Part print with two shaded views. Sizes in mm from the minimum x, y, z corner. Coordinates: 2 decimals unless noted, no trailing zeros. Loops run counter-clockwise (first coordinate to the right, second up) from the corner with the lowest first, then second, coordinate; pieces in that order, holes last. Notation, with made-up numbers: (-11.5, 9) - (27.5, 9) arc R15 ccw to (27.5, 29) - close; hole circle Ø2 at (72, 86). An arc over 180 degrees is marked (long way). Answer as CSV lines item,"result".
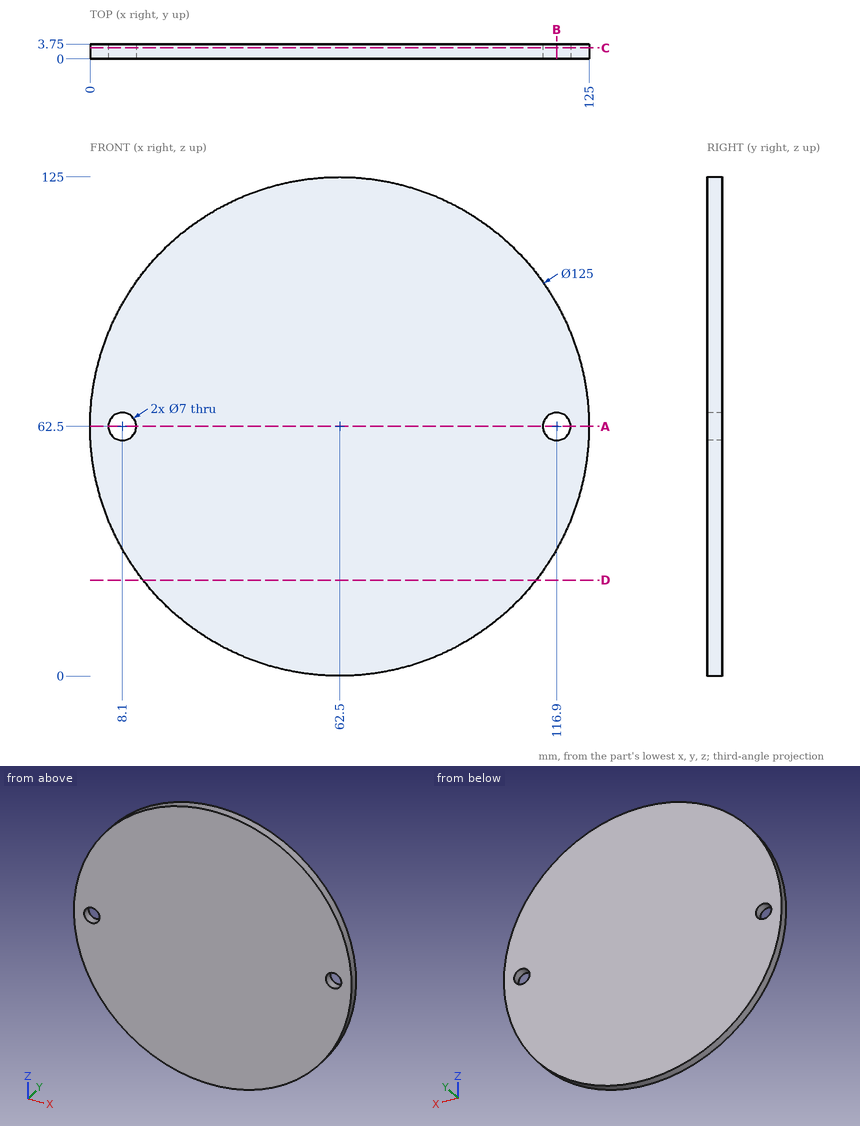
Q1. Saw through at C-C (y = 2.75). Give the cut face in (x, z).
Results:
outline,"circle Ø125 at (62.5, 62.5); hole circle Ø7 at (8.1, 62.5); hole circle Ø7 at (116.9, 62.5)"
Q2. Flat gauge pins, fed straight in: pin 1 (2 mm diameter, centred on y = 3, z = 29.5, fed in from +X); pin 2 (5.5 mm diameter, centred on x = 116.9, z = 62.5, fed in from -Y). Where does each tip first touch, or does it go through?
Results:
pin 1,"stops at x = 116.19"
pin 2,"passes through"
Q3. Saw through at B-B (x = 116.9). Give the cut face in (y, z).
Results:
outline,"(0, 31.73) - (3.75, 31.73) - (3.75, 59) - (0, 59) - close; (0, 66) - (3.75, 66) - (3.75, 93.27) - (0, 93.27) - close"
Q4. Wall check: L1, parallel to Z at x = 116.9, y = 1.3; L2, parallel to Z at x = 118, y = 1.15; L3, parallel to Z at x = 12, y = 0.6. Give the ranges that are in metal, low to high.
Results:
L1,"z = 31.73 to 59, 66 to 93.27"
L2,"z = 33.76 to 59.18, 65.82 to 91.24"
L3,"z = 25.68 to 99.32"
Q5. Saw through at D-D (z = 24). Give the cut face in (x, y).
Results:
outline,"(13.27, 0) - (111.73, 0) - (111.73, 3.75) - (13.27, 3.75) - close"
Q6. Saw through at A-A (z = 62.5). Give the cut face in (x, y).
Results:
outline,"(0, 0) - (4.6, 0) - (4.6, 3.75) - (0, 3.75) - close; (11.6, 0) - (113.4, 0) - (113.4, 3.75) - (11.6, 3.75) - close; (120.4, 0) - (125, 0) - (125, 3.75) - (120.4, 3.75) - close"
